Source: CAD feature listing. Evaluate the final solid. Frame: model axes, mm. A direction names the side the tool comes from. Round coordinates to 2 decimals unless told otherwise and drop trailing zeros. Loops run counter-clockwise (first coordinate to the right, second up) from the corner with the lowest first, then second, coordinate; pieces in that order, holes last.
Item 1: Section query B-B on x = 27. Return loops of the section in (y, z), then the cut area to 3 significant figures.
Item 2: First-contact query: P1, Ø1.8, axis at x = 4, y = 0.5, coming from the -Z side; P2, Ø1.5, axis at x = 44, z = -16.5, coming from the +Y side; P3, Ø0.5, axis at x = 7, y = 1, coming from the +Z side. Flat tips, straight axial feed; report the tip coordinate or a pass-through.
Item 3: Pull-direction query (X, two-part tool) for faces 1 (the flat face through (3, 1, 18.8)), 2 (the cylindrical face through (64.55, 0.81, 18.37)), 3 (the flat face through (9, 1, -17.8)); classes: released by +X, released by -X, zero draft, split by the parting line, or undercut.
Item 4: Section query C-C on z = -1.5. Return loops of the section in (x, y).
Item 5: Ray query, L1, parallel to Y at x = 54.5, z = 17; L2, parallel to Z at x = 31.5, y = 0.25; L3, parallel to Y at x = 5.5, z = 4.5. Return the intervals inside material, ascending.
Item 6: Access query for faces 4 (the flat face through (9, 1, 16.8)), 5 (the flat face through (37, 1, 18.8)), 6 (the flat face through (37, 1, -18.8)). Directions: +Z, -Z, +X, -X, +Y, -Y. A direction counts if a zero-diameter tool reaches every point of the face in a straight line with its end or side. Return the directions, or none.
Item 7: Section query D-D on z = 4.5. Return loops of the section in (x, y), then the cut area to 3 significant figures.
Item 8: Section query A-A on x = 9.5. Return loops of the section in (y, z), then the cut area to 3 significant figures.
```python
from build123d import *

# Parameters (mm, degrees)
BOSS_EXTRUDE1_DEPTH      = 65
SKETCH2_R                = 4.4
BOSS_EXTRUDE_LATCH_DEPTH = 1.6
SKETCH3_W                = 11
SKETCH3_H                = 1
CUT_EXTRUDE1_DEPTH       = 68.880851497
FILLET1_R                = 1.5


with BuildPart() as part:
    # Sketch1 → Boss-Extrude1 (new body)
    with BuildSketch(Plane(origin=(0, 0, 0), x_dir=(0, 0, -1), z_dir=(1, 0, 0))):
        Polygon((18.8, 0), (-18.8, 0), (-18.8, 1.6), (-16.8, 1.6), (-15.3, 3), (15.3, 3), (16.8, 1.6), (18.8, 1.6), align=None)
    extrude(amount=BOSS_EXTRUDE1_DEPTH)

    # Sketch2 → Boss-Extrude-Latch (add)
    with BuildSketch(Plane(origin=(0, 1.6, 0), x_dir=(1, 0, 0), z_dir=(0, 1, 0))):
        with Locations((9, 15.1)):
            Circle(SKETCH2_R)
        with Locations((9, -15.1)):
            Circle(SKETCH2_R)
    extrude(amount=-BOSS_EXTRUDE_LATCH_DEPTH)

    # Sketch3 → Cut-Extrude1 (cut, through all)
    with BuildSketch(Plane(origin=(0, 1.6, 0), x_dir=(1, 0, 0), z_dir=(0, 1, 0))):
        with Locations((9, 17.3)):
            Rectangle(SKETCH3_W, SKETCH3_H)
        with Locations((9, -17.3)):
            Rectangle(SKETCH3_W, SKETCH3_H)
    extrude(amount=-CUT_EXTRUDE1_DEPTH, mode=Mode.SUBTRACT)

    # Sketch4 → Cut-Revolve1 (revolve, cut)
    with BuildSketch(Plane.XY):
        with BuildLine():
            Line((12, 39.818181818), (12, 0.8))
            ThreePointArc((12, 0.8), (-7.509090909, 20.309090909), (12, 39.818181818))
        make_face()
    revolve(axis=Axis((12, 39.818181818, 0), (0, -1, 0)), mode=Mode.SUBTRACT)

    # Fillet1
    fillet1_edges = [part.edges().sort_by_distance(p)[0] for p in [
        (65, 0.8, -18.8),
        (65, 2.3, -16.05),
        (65, 2.3, 16.05),
        (65, 0.8, 18.8),
    ]]
    fillet(fillet1_edges, radius=FILLET1_R)


solid = part.part
```
Data:
1. outline: (0, -18.8) - (1.6, -18.8) - (1.6, -16.8) - (3, -15.3) - (3, 15.3) - (1.6, 16.8) - (1.6, 18.8) - (0, 18.8) - close
1. area: 105 mm2
2. P1: stops at z = -18.8
2. P2: stops at y = 2.58
2. P3: stops at z = 19.14
3. face 1: zero draft
3. face 2: released by +X
3. face 3: undercut
4. outline: (0, 0) - (65, 0) - (65, 3) - (20.87, 3) arc R19.45 cw to (3.13, 3) - (0, 3) - close
5. L1: y = 0 to 1.6
5. L2: z = -18.8 to 18.8
5. L3: y = 0 to 2.47
6. face 4: +Y, -Y
6. face 5: +Z, +X, +Y, -Y
6. face 6: -Z, +X, +Y, -Y
7. outline: (0, 0) - (65, 0) - (65, 3) - (19.79, 3) arc R18.98 cw to (4.21, 3) - (0, 3) - close
7. area: 177 mm2
8. outline: (0, -19.47) - (1.6, -19.47) - (1.6, -17.8) - (0, -17.8) - close; (0, -16.8) - (1.6, -16.8) - (3, -15.3) - (3, -8.65) arc R19.35 cw to (3, 8.65) - (3, 15.3) - (1.6, 16.8) - (0, 16.8) - close; (0, 17.8) - (1.6, 17.8) - (1.6, 19.47) - (0, 19.47) - close
8. area: 80.3 mm2
